from build123d import *

# Parameters (mm, degrees)
SKETCH_1_W             = 220
SKETCH_1_H             = 7
EXTRUDE_1_DEPTH        = 2
PATTERN_LINEAR_2_COUNT = 10
PATTERN_LINEAR_2_PITCH = 7


with BuildPart() as part:
    # 草图1 → 凸台-拉伸1 (new body)
    with BuildSketch(Plane.XY):
        Rectangle(SKETCH_1_W, SKETCH_1_H)
    extrude(amount=EXTRUDE_1_DEPTH)

    # 草图6 → M3 螺纹孔2 (revolve, cut)
    with BuildSketch(Plane(origin=(-106, 0, 2), x_dir=(0, -1, 0), z_dir=(1, 0, 0))):
        Polygon((0, 0), (0, 8.251075774), (1.25, 7.5), (1.25, 0), align=None)
    hole_wizard_m3_2 = revolve(axis=Axis((-106, 0, 8.35), (0, 0, -1)), mode=Mode.SUBTRACT)

    # 阵列(线性)2: M3 螺纹孔2 ×10
    with Locations(*[(i * PATTERN_LINEAR_2_PITCH, 0, 0) for i in range(1, PATTERN_LINEAR_2_COUNT)]):
        add(hole_wizard_m3_2, mode=Mode.SUBTRACT)

    # 镜向1: M3 螺纹孔2 across plane
    add(hole_wizard_m3_2.mirror(Plane(origin=(0, 0, 0), x_dir=(0, 0, 1), z_dir=(1, 0, 0))), mode=Mode.SUBTRACT)

    # 镜向1 copy 1 sketch → 镜向1 copy 1 (revolve, cut)
    with BuildSketch(Plane(origin=(99, 0, 2), x_dir=(0, -1, 0), z_dir=(-1, 0, 0))):
        Polygon((0, 0), (0, -8.251075774), (1.25, -7.5), (1.25, 0), align=None)
    revolve(axis=Axis((99, 0, 8.35), (0, 0, 1)), mode=Mode.SUBTRACT)

    # 镜向1 copy 2 sketch → 镜向1 copy 2 (revolve, cut)
    with BuildSketch(Plane(origin=(92, 0, 2), x_dir=(0, -1, 0), z_dir=(-1, 0, 0))):
        Polygon((0, 0), (0, -8.251075774), (1.25, -7.5), (1.25, 0), align=None)
    revolve(axis=Axis((92, 0, 8.35), (0, 0, 1)), mode=Mode.SUBTRACT)

    # 镜向1 copy 3 sketch → 镜向1 copy 3 (revolve, cut)
    with BuildSketch(Plane(origin=(85, 0, 2), x_dir=(0, -1, 0), z_dir=(-1, 0, 0))):
        Polygon((0, 0), (0, -8.251075774), (1.25, -7.5), (1.25, 0), align=None)
    revolve(axis=Axis((85, 0, 8.35), (0, 0, 1)), mode=Mode.SUBTRACT)

    # 镜向1 copy 4 sketch → 镜向1 copy 4 (revolve, cut)
    with BuildSketch(Plane(origin=(78, 0, 2), x_dir=(0, -1, 0), z_dir=(-1, 0, 0))):
        Polygon((0, 0), (0, -8.251075774), (1.25, -7.5), (1.25, 0), align=None)
    revolve(axis=Axis((78, 0, 8.35), (0, 0, 1)), mode=Mode.SUBTRACT)

    # 镜向1 copy 5 sketch → 镜向1 copy 5 (revolve, cut)
    with BuildSketch(Plane(origin=(71, 0, 2), x_dir=(0, -1, 0), z_dir=(-1, 0, 0))):
        Polygon((0, 0), (0, -8.251075774), (1.25, -7.5), (1.25, 0), align=None)
    revolve(axis=Axis((71, 0, 8.35), (0, 0, 1)), mode=Mode.SUBTRACT)

    # 镜向1 copy 6 sketch → 镜向1 copy 6 (revolve, cut)
    with BuildSketch(Plane(origin=(64, 0, 2), x_dir=(0, -1, 0), z_dir=(-1, 0, 0))):
        Polygon((0, 0), (0, -8.251075774), (1.25, -7.5), (1.25, 0), align=None)
    revolve(axis=Axis((64, 0, 8.35), (0, 0, 1)), mode=Mode.SUBTRACT)

    # 镜向1 copy 7 sketch → 镜向1 copy 7 (revolve, cut)
    with BuildSketch(Plane(origin=(57, 0, 2), x_dir=(0, -1, 0), z_dir=(-1, 0, 0))):
        Polygon((0, 0), (0, -8.251075774), (1.25, -7.5), (1.25, 0), align=None)
    revolve(axis=Axis((57, 0, 8.35), (0, 0, 1)), mode=Mode.SUBTRACT)

    # 镜向1 copy 8 sketch → 镜向1 copy 8 (revolve, cut)
    with BuildSketch(Plane(origin=(50, 0, 2), x_dir=(0, -1, 0), z_dir=(-1, 0, 0))):
        Polygon((0, 0), (0, -8.251075774), (1.25, -7.5), (1.25, 0), align=None)
    revolve(axis=Axis((50, 0, 8.35), (0, 0, 1)), mode=Mode.SUBTRACT)

    # 镜向1 copy 9 sketch → 镜向1 copy 9 (revolve, cut)
    with BuildSketch(Plane(origin=(43, 0, 2), x_dir=(0, -1, 0), z_dir=(-1, 0, 0))):
        Polygon((0, 0), (0, -8.251075774), (1.25, -7.5), (1.25, 0), align=None)
    revolve(axis=Axis((43, 0, 8.35), (0, 0, 1)), mode=Mode.SUBTRACT)


solid = part.part
Can you work these out from the model? Positions are in its coordinate system, mm. Round coordinates to 2 decimals unless told otherwise and drop trailing zeros. Write each question's results on one line, items separated by ' | '. Start each with the question number.
Item 1: Will these pins go through, and if not, where does the flat tip stop? pin 1 (1.5 mm diameter, centred on x = 106, y = 0, fed in from -Z); pin 2 (3 mm diameter, centred on x = -99, y = 0, fed in from -Z).
Item 2: If we section it at A-A, the plane z = 1.35: State how many separate pieces and enclosed holes the cut face has, then the cut area to 3 significant figures.
Item 3: Please list where these lines run through material, in increasing order: L1, parallel to Y at x = 71, z = 1; L2, parallel to Y at x = 84.5, z = 0.8.
Results:
1) pin 1: passes through | pin 2: stops at z = 0
2) separate pieces: 1 | enclosed holes: 20 | area: 1,440 mm2
3) L1: y = -3.5 to -1.25, 1.25 to 3.5 | L2: y = -3.5 to -1.15, 1.15 to 3.5
